Autodesk Inventor part; units mm, degrees
ref_plane "YZ Plane" through (0, 0, 0) normal (1, 0, 0) x (0, 1, 0)
ref_plane "XZ Plane" through (0, 0, 0) normal (0, 1, 0) x (-1, 0, 0)
ref_plane "XY Plane" through (0, 0, 0) normal (0, 0, 1) x (1, 0, 0)
sketch "Sketch1" plane through (0, 0, 0) normal (0, 1, 0) x (-1, 0, 0)
  circle A0 centre (0, 0) radius 29
  dimension "d0" = 58
extrude "Extrusion1" add sketch "Sketch1" along normal blind 4
sketch "Sketch2" plane through (0, 4, 0) normal (0, 1, 0) x (1, 0, 0)
  circle A0 centre (0, 0) radius 15.5
  dimension "d3" = 31
extrude "Extrusion2" cut sketch "Sketch2" against normal through all
sketch "Sketch3" plane through (0, 4, 0) normal (0, 1, 0) x (1, 0, 0)
  circle A0 centre (-24.5, 0) radius 2
  point P0 (0, 0)
  dimension "d6" = 24.5
  dimension "d7" = 4
extrude "Extrusion3" cut sketch "Sketch3" against normal through all
sketch "Sketch4" plane through (0, 4, 0) normal (0, 1, 0) x (1, 0, 0)
  line L0 (10, -34.3438) -> (33.4765, -34.3438)
  line L1 (33.4765, -34.3438) -> (33.4765, 39.4177)
  line L2 (33.4765, 39.4177) -> (10, 39.4177)
  line L3 (10, 39.4177) -> (10, -34.3438)
  point P0 (0, 0)
  dimension "d13" = 10
extrude "Extrusion4" cut sketch "Sketch4" against normal blind 10
sketch "Sketch5" plane through (0, 0, 0) normal (0, 0, 1) x (1, 0, 0)
  line L0 (10, 4) -> (-29, 4)
  line L1 (10, 4) -> (20.1905, 24)
  line L2 (10, 4) -> (32.4465, 4) construction
  line L3 (20.1905, 24) -> (17.1905, 24)
  line L4 (17.1905, 24) -> (7, 4)
  line L5 (7, 4) -> (10, 4)
  line L6 (10, 0) -> (10, 4)
  line L7 (10, 4) -> (10, 0)
  line L8 (7, 4) -> (4.9619, 0)
  line L9 (10, 0) -> (-15.5, 0)
  line L10 (4.9619, 0) -> (10, 0)
  point P0 (0, 0)
  point P1 (7, 4)
  point P2 (18.6905, 24)
  dimension "d16" = 63
  dimension "d17" = 3
  dimension "d18" = 117
  dimension "d21" = 20
extrude "Extrusion5" add sketch "Sketch5" along normal mid plane 50 contours L0 L4 L3 L1
sketch "Sketch6" plane through (7, 4, -25) normal (-0.891, 0.454, 0) x (0, 0, 1)
  line L0 (11.1707, 0) -> (38.8293, 0)
  line L1 (15, 2) -> (29, 2)
  line L2 (29, 2) -> (29, 18.4465)
  line L3 (29, 18.4465) -> (15, 18.4465)
  line L4 (15, 18.4465) -> (15, 2)
  line L5 (50, 22.4465) -> (0, 22.4465)
  point P0 (25, -6.742)
  point P1 (25, 0)
  point P2 (25, 0)
  point P3 (40, 22.4465)
  point P4 (10, 22.4465)
  dimension "d37" = 4
  dimension "d38" = 10
  dimension "d39" = 4
  dimension "d40" = 2
extrude "Extrusion6" cut sketch "Sketch6" against normal blind 46
sketch "Sketch7" plane through (7, 4, -25) normal (-0.891, 0.454, 0) x (0, 0, 1)
  circle A0 centre (9, 13) radius 1.5
  circle A1 centre (41, 13) radius 1.5
  line L0 (50, 0) -> (38.8293, 0)
  line L1 (11.1707, 0) -> (0, 0)
  ellipse E0 centre (25, -14.3007) end of major axis (27, -14.3007) minor radius 0.908
  point P0 (25, -6.742)
  dimension "d29" = 3
  dimension "d30" = 3
  dimension "d31" = 13
  dimension "d32" = 13
  dimension "d46" = 16
  dimension "d47" = 16
extrude "Extrusion7" cut sketch "Sketch7" against normal blind 46 contours A0 | A1
sketch "Sketch8" plane through (0, 0, 25) normal (0, 0, 1) x (1, 0, 0)
  line L0 (10, 4) -> (10, 0)
  line L1 (10, 4) -> (10, 0)
  line L2 (10, 4) -> (-29, 4)
  line L3 (7, 4) -> (4.9619, 0)
  line L4 (10, 0) -> (-29, 0)
  line L5 (7, 4) -> (11.4893, 4) construction
  line L6 (4.9619, 0) -> (10, 0)
  point P0 (0, 0)
  dimension "d43" = 117
extrude "Extrusion8" add sketch "Sketch8" against normal blind 46
properties part number "Nose cam retention"
Geometry: final body of the model. Coordinates: model frame, mm. A direction names the side the tool comes from. Round coordinates to 2 decimals unless told otherwise and drop trailing zeros. Order: outer loops, then holes, each group sorted by start corner. A loop starts at its lowest first (then second) coordinate and runs counter-clockwise, first axis right, second up. Notation, with made-up numbers: (-4, 53) -> (3, 53) arc R21 ccw to (3, 70) -> close; hole circle Ø7 at (-20.75, 23). An arc over 180 degrees is marked (long way). Use CSV: the item, a comma, the result in double quotes. Start each with the question number.
1) Draft query along Z for faces 4 (the face through (14, 14, 25)), 5 (the face through (-26.498, 2.028, -0.088)), 6 (the face through (19, 24, 0)). Return one class per face: +Z half, -Z half, draft (parallel to the pull), parting line (faces both ways), or undercut.
2) Section B-B (x = 0). Return the cut outline in (y, z), and give its area (3 significant figures).
3) Section C-C (y = 18.5). Return the cut outline in (x, z), and give its area (3 significant figures).
4) Material intervals for line 1 along Z through (x, y) = (-24.5, 1.2); line 2 along X through (y, z) = (1.75, 0); line 3 along Z through (x, y) = (0, 2.9), sorted ascending. Write a range as from..to.
5) First-contact query: pin 1 Ø6.5 at (x, y) = (10.5, 14.5) entering from +Z; pin 2 Ø1 at (y, z) = (6, 2.5) entering from +X; pin 3 Ø5 at (x, y) = (14.5, 10) entering from -Z. Flat tips, straight axial feed; report the tip coordinate or a pass-through.
6) Section A-A (z = 0). Return the cut outline in (x, y).
7) Section D-D (z = -6). Return the cut outline in (x, y).
8) Set-up query: faces 1 (the face through (9.082, 5.184, -3.098)), 2 (the face through (14, 14, -25)), 3 (the face through (16.549, 19.838, -2.902)). Return all of +Z, -Z, +X, -X, +Y, -Y with unobstructed straight access to the full face (end or side cutting, diameter ignored); none if empty.
Returned:
1,face 4,"+Z half"
1,face 5,"undercut"
1,face 6,"draft"
2,outline,"(0, -29) -> (4, -29) -> (4, -15.5) -> (0, -15.5) -> close; (0, 15.5) -> (4, 15.5) -> (4, 29) -> (0, 29) -> close"
2,area,"108 mm²"
3,outline,"(14.39, -25) -> (17.39, -25) -> (17.39, -10) -> (14.39, -10) -> close; (14.39, 4) -> (17.39, 4) -> (17.39, 25) -> (14.39, 25) -> close"
3,area,"108 mm²"
4,line 1,"z = -15.52..-2, 2..15.52"
4,line 2,"x = -29..-26.5, -22.5..-15.5, 5.85..10"
4,line 3,"z = -29..-15.5, 15.5..29"
5,pin 1,"stops at z = 25"
5,pin 2,"stops at x = 8.46"
5,pin 3,"stops at z = -25"
6,outline,"(-29, 0) -> (-26.5, 0) -> (-26.5, 4) -> (-29, 4) -> close; (-22.5, 0) -> (-15.5, 0) -> (-15.5, 4) -> (-22.5, 4) -> close; (4.96, 0) -> (10, 0) -> (10, 4) -> (10.29, 4.57) -> (7.91, 5.78) -> close; (15.37, 20.44) -> (17.76, 19.22) -> (20.19, 24) -> (17.19, 24) -> close"
7,outline,"(-28.37, 0) -> (-14.29, 0) -> (-14.29, 4) -> (-28.37, 4) -> close; (4.96, 0) -> (10, 0) -> (10, 4) -> (10.29, 4.57) -> (7.91, 5.78) -> close; (15.37, 20.44) -> (17.76, 19.22) -> (20.19, 24) -> (17.19, 24) -> close"
8,face 1,"+X, +Y"
8,face 2,"-Z, +X, -X, +Y"
8,face 3,"-X, -Y"
